```python
from build123d import *

# Parameters (mm, degrees)
F0_W     = 600
F0_H     = 1200
F1_DEPTH = 75
F2_W     = 600
F2_H     = 1200
F2_W_2   = 590
F2_H_2   = 620
F2_H_3   = 565
F3_DEPTH = 2
F4_W     = 96
F4_H     = 1030
F5_DEPTH = 75


# Not quite as in the source:
# - a pattern or mirror of a feature is missing from the dataset's text; its kind, count and spacing are read off the source's solid


with BuildPart() as f1:
    # F0 (on Front) → F1 (new body, symmetric)
    with BuildSketch(Plane.XZ):
        with Locations((-546.9189941883, 533.8190406561)):
            Rectangle(F0_W, F0_H)
    extrude(amount=F1_DEPTH, both=True)

    # F2 (on face) → F3 (cut)
    with BuildSketch(Plane.XZ.offset(75)):
        with Locations((-546.9189941883, 533.8190406561)):
            Rectangle(F2_W, F2_H)
        with Locations((-546.9189941883, 248.8190406561)):
            Rectangle(F2_W_2, F2_H_2, mode=Mode.SUBTRACT)
        with Locations((-546.9189941883, 846.3190406561)):
            Rectangle(F2_W_2, F2_H_3, mode=Mode.SUBTRACT)
    f3 = extrude(amount=-F3_DEPTH, mode=Mode.SUBTRACT)

    # F3_copies: F3 across plane
    add(f3.mirror(Plane.ZX), mode=Mode.SUBTRACT)

    # F4 (on face) → F5 (join)
    with BuildSketch(Plane(origin=(-846.9189941883, 0, 0), x_dir=(0, -1, 0), z_dir=(-1, 0, 0))):
        with Locations((0, 533.8190406561)):
            Rectangle(F4_W, F4_H)
    extrude(amount=F5_DEPTH)


solid = f1.part
```
The listing builds one solid part. Answer for the finished solid, in the listing's coordinates (mm). A direction names the side the tool comes from. Round coordinates to 2 decimals unless told otherwise and drop trailing zeros. Loops run counter-clockwise (first coordinate to the right, second up) from the corner with the lowest first, then second, coordinate; pieces in that order, holes last. Notation, with made-up numbers: (-12.5, 48) -> (26.5, 48) arc R14 cw to (26.5, 64) -> close; hole circle Ø4 at (-37, 46.5). An arc over 180 degrees is marked (long way). Use one line per item in the form item = value.
1. The part is cut by section A-A on y = 21. Determine the outline of the cut face in (x, z), and give its area (3 significant figures).
Answer key:
outline = (-921.92, 18.82) -> (-846.92, 18.82) -> (-846.92, -66.18) -> (-246.92, -66.18) -> (-246.92, 1133.82) -> (-846.92, 1133.82) -> (-846.92, 1048.82) -> (-921.92, 1048.82) -> close
area = 797,000 mm²
2. The part is cut by section B-B on z = 629. Determine the outline of the cut face in (x, y).
Answer key:
outline = (-921.92, -48) -> (-846.92, -48) -> (-846.92, -73) -> (-841.92, -73) -> (-841.92, -75) -> (-251.92, -75) -> (-251.92, -73) -> (-246.92, -73) -> (-246.92, 73) -> (-251.92, 73) -> (-251.92, 75) -> (-841.92, 75) -> (-841.92, 73) -> (-846.92, 73) -> (-846.92, 48) -> (-921.92, 48) -> close
3. A tool of negligible diameter and unlimited length cuts with its end or side. For faces 1 (the flat face through (-884, 1, 1048.819)), 2 (the flat face through (-884, 48, 527)), 3 (the flat face through (-884, 1, 18.819)), from which of +Z, -Z, +X, -X, +Y, -Y can it reach the whole face along a straight path? Write none if from no direction.
Answer key:
face_1 = +Z, -X, +Y, -Y
face_2 = +Z, -Z, -X, +Y
face_3 = -Z, -X, +Y, -Y
4. Flat-ended cylindrical pins translate along their axes: pin 1 Ø22.5 at (x, z) = (-886.5, 754) entering from +Y; pin 2 Ø2 at (y, z) = (-74.5, 280) entering from +X; pin 3 Ø1.6 at (y, z) = (74.5, 130.5) entering from -X. Find the tip coordinate at first contact, or state that the pin passes through.
Answer key:
pin_1 = 48
pin_2 = -251.92
pin_3 = -841.92
5. Find the intervals of material crossed by probe 1 along X at (y, z) = (-55, 592.5), in increasing order. Write a range as [from, to].
Answer key:
probe_1 = [-846.92, -246.92]
